Input: part model. Units: mm. Frame: model coordinates. Face numbers are marked on the shaded views. A direction names the side the tool comes from. Coordinates: 2 decimals unless noted, no trailing zeros. Write each loop counter-clockwise with the first axis right and the second up, starting at its lowest first coordinate (ties: lowest second). Pieces come first, ordered by that corner, then holes. Notation, with made-up numbers: M 61,39 L 81,39 A11 ccw 81,50 Z; hole C -1,49.5 d11. An arc over 180 degrees is marked long. Answer as a JSON object with one key per item and string values. Group by question number.
from build123d import *

# Parameters (mm, degrees)
ESBO_O1_R                     = 40
ESBO_O1_R_2                   = 30
RESSALTO_EXTRUS_O1_DEPTH      = 50
ESBO_O2_R                     = 1.5
CORTE_EXTRUS_O1_DEPTH         = 6
CORTE_EXTRUS_O2_DEPTH         = 11.84997677
RESSALTO_EXTRUS_O2_DEPTH      = 26.84997677
RESSALTO_EXTRUS_O2_DEPTH_BACK = 10
REVOLU_O1_ANGLE               = 180
RESSALTO_EXTRUS_O5_DEPTH      = 5
RESSALTO_EXTRUS_O5_DEPTH_BACK = 2
ESBO_O10_R                    = 11
ESBO_O13_R                    = 8
CORTE_EXTRUS_O4_DEPTH         = 40


# Read off the part's stored shape, not the designer's step: Limites1
with BuildPart() as part:
    # Esboço1 → Ressalto-extrusão1 (new body)
    with BuildSketch(Plane(origin=(0, 0, 0), x_dir=(1, 0, 0), z_dir=(0, 1, 0))):
        with Locations(Location((0, 0, 0), (0, 0, 270))):
            Circle(ESBO_O1_R)
        with Locations(Location((0, 0, 0), (0, 0, 270))):
            Circle(ESBO_O1_R_2, mode=Mode.SUBTRACT)
    extrude(amount=RESSALTO_EXTRUS_O1_DEPTH)

    # Esboço2 → Corte-extrusão1 (cut)
    with BuildSketch(Plane(origin=(0, 0, 0), x_dir=(-1, 0, 0), z_dir=(0, -1, 0))):
        with Locations(Location((-21.160269083, -29.124611797, 0), (0, 0, 90))):
            Circle(ESBO_O2_R)
        with Locations(Location((-34.238034587, -11.124611797, 0), (0, 0, 90))):
            Circle(ESBO_O2_R)
        with Locations(Location((-34.238034587, 11.124611797, 0), (0, 0, 90))):
            Circle(ESBO_O2_R)
        with Locations(Location((21.160269083, 29.124611797, 0), (0, 0, 90))):
            Circle(ESBO_O2_R)
        with Locations(Location((34.238034587, 11.124611797, 0), (0, 0, 90))):
            Circle(ESBO_O2_R)
        with Locations(Location((34.238034587, -11.124611797, 0), (0, 0, 90))):
            Circle(ESBO_O2_R)
    extrude(amount=-CORTE_EXTRUS_O1_DEPTH, mode=Mode.SUBTRACT)

    # Esboço3 → Corte-extrusão2 (cut)
    with BuildSketch(Plane(origin=(0, 0, 0), x_dir=(-1, 0, 0), z_dir=(0, -1, 0))):
        with BuildLine():
            ThreePointArc((30.293924668, -13.087327008), (31.253408489, 10.593604572), (16.092357529, 28.81034587))
            Line((16.092357529, 28.81034587), (19.505887914, 34.921631358))
            ThreePointArc((19.505887914, 34.921631358), (8.030354378, 39.185627576), (-4.197370073, 39.779166463))
            Line((-4.197370073, 39.779166463), (-3.148027555, 29.834374847))
            ThreePointArc((-3.148027555, 29.834374847), (29.911212101, 2.306380417), (1.462902849, -29.964310692))
            Line((1.462902849, -29.964310692), (1.950537132, -39.952414256))
            ThreePointArc((1.950537132, -39.952414256), (22.185986252, -33.283359416), (36.126859334, -17.171197823))
            Line((36.126859334, -17.171197823), (30.293924668, -13.087327008))
        make_face()
    extrude(amount=-CORTE_EXTRUS_O2_DEPTH, mode=Mode.SUBTRACT)

    # Esboço4 → Ressalto-extrusão2 (add, two sides: drawn at the far end of the back side and taken through both)
    with BuildSketch(Plane(origin=(0, 11.84997677, 0), x_dir=(-1, 0, 0), z_dir=(0, -1, 0)).offset(-RESSALTO_EXTRUS_O2_DEPTH_BACK)):
        with BuildLine():
            Line((-4.008838629, -29.730947056), (-4.700362463, -27.602655537))
            ThreePointArc((-4.700362463, -27.602655537), (-8.119302432, 26.79695744), (19.230258499, -20.351834268))
            Line((19.230258499, -20.351834268), (19.909240802, -22.441526924))
            ThreePointArc((19.909240802, -22.441526924), (-8.745833796, 28.696870757), (-4.008838629, -29.730947056))
        make_face()
    extrude(amount=RESSALTO_EXTRUS_O2_DEPTH + RESSALTO_EXTRUS_O2_DEPTH_BACK)

    # Esboço9 → Revolução1 (revolve)
    with BuildSketch(Plane(origin=(0, 50, 0), x_dir=(1, 0, 0), z_dir=(0, 1, 0))):
        with BuildLine():
            Line((-40, 0), (-30, 0))
            ThreePointArc((-30, 0), (0, 30), (30, 0))
            Line((30, 0), (40, 0))
            ThreePointArc((40, 0), (0, 40), (-40, 0))
        make_face()
    revolve(axis=Axis((-40, 50, 0), (1, 0, 0)), revolution_arc=REVOLU_O1_ANGLE)

    # Esboço10 → Ressalto-extrusão5 (add, two sides: drawn at the far end of the back side and taken through both)
    with BuildSketch(Plane(origin=(0, 90, 0), x_dir=(1, 0, 0), z_dir=(0, 1, 0)).offset(-RESSALTO_EXTRUS_O5_DEPTH_BACK)):
        with Locations(Location((0, 0, 0), (0, 0, 270))):
            Circle(ESBO_O10_R)
    extrude(amount=RESSALTO_EXTRUS_O5_DEPTH + RESSALTO_EXTRUS_O5_DEPTH_BACK)

    # Limites1 outline → Limites1 (revolve)
    with BuildSketch(Plane.XY):
        Polygon((11, 95), (10.5, 115), (0, 115), (0, 95), align=None)
    revolve(axis=Axis((0, 0, 0), (0, 1, 0)))

    # Esboço13 → Corte-extrusão4 (cut)
    with BuildSketch(Plane(origin=(0, 115, 0), x_dir=(1, 0, 0), z_dir=(0, 1, 0))):
        with Locations(Location((0, 0, 0), (0, 0, 270))):
            Circle(ESBO_O13_R)
    extrude(amount=-CORTE_EXTRUS_O4_DEPTH, mode=Mode.SUBTRACT)


solid = part.part
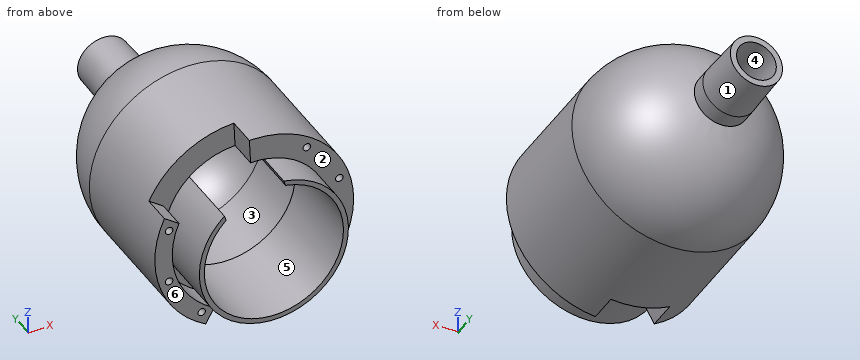
Q1. Section A-A, the plane z = 0. Return the cut outline in (x, y).
Q2. Section D-D, the plane z = -32.5. Return the cut outline in (x, y), and give its area (3 significant figures).
Q3. Section C-C, the plane y = 29. Return the cut outline in (x, z), and give its area (3 significant figures).
Q4. Pin query (flat end, axial travel): pin 1 Ø2.5 at (x, z) = (33.5, -12) entering from -Y; pin 2 Ø1.5 at (x, y) = (15.5, 63) entering from -Z; pin 3 Ø3 at (y, z) = (64.5, -12) entering from -X (3 decimals); pin 4 Ø14.5 at (x, z) = (0, 0) entering from -Y. Return the tip coordinate at first contact, or that it passes through.
Q5. Section B-B, the plane x = 0. Return the cut outline in (y, z), and give its area (3 significant figures).
Q6. Access query for the marked faces 4, 5 and 6. Directions: +Z, -Z, +X, -X, +Y, -Y. A direction counts if a zero-diameter tool reaches every point of the face in a straight line with its end or side. Return the directions, or none.
Q7. Draft query along Y for the marked faces 1, 2 and 3. Return one class per face: released by +Y, released by -Y, zero draft, split by the parting line, or undercut.
Q8. Line query: line 1 (X direction, y = 1.5, z = 0); line 2 (X direction, y = 17, z = -11); line 3 (Z direction, x = 5.5, y = 106.5). Output: solid intervals per line, ascending. Write a range as from..to.
Filled in:
{
 "1": {"outline": "M -40,0 L -33,0 L -33,11.85 L -30,11.85 L -30,-15 L -28,-15 L -28,21.85 L -30,21.85 L -30,50 A30 cw -8,78.91 L -8,115 L -10.5,115 L -11,95 L -11,88.46 A40 ccw -40,50 Z; M 8,78.91 A30 cw 30,50 L 30,21.85 L 28,21.85 L 28,-15 L 30,-15 L 30,0 L 40,0 L 40,50 A40 ccw 11,88.46 L 11,95 L 10.5,115 L 8,115 Z"},
 "2": {"outline": "M -23.32,0 L -18.15,0 L -18.15,11.85 L 3.43,11.85 L 3.43,0 L 23.32,0 L 23.32,50 A23.32 ccw -23.32,50 Z", "area": "2,930 mm^2"},
 "3": {"outline": "C 0,0 d80; hole C 0,0 d60", "area": "2,200 mm^2"},
 "4": {"pin 1": "y = 0", "pin 2": "z = -34.94", "pin 3": "x = -36.055", "pin 4": "through"},
 "5": {"outline": "M -15,-30 L 11.85,-30 L 11.85,-40 L 50,-40 A40 ccw 88.46,-11 L 95,-11 L 115,-10.5 L 115,-8 L 78.91,-8 A30 cw 50,-30 L 21.85,-30 L 21.85,-28 L -15,-28 Z; M 0,30 L 50,30 A30 cw 78.91,8 L 115,8 L 115,10.5 L 95,11 L 88.46,11 A40 ccw 50,40 L 0,40 Z", "area": "2,040 mm^2"},
 "6": {"face 4": "+Y, -Y", "face 5": "-Y", "face 6": "-Z, -X, -Y"},
 "7": {"face 1": "released by +Y", "face 2": "released by -Y", "face 3": "undercut"},
 "8": {"line 1": "-40..-33, -30..-28, 28..40", "line 2": "-38.46..-25.75, 25.75..38.46", "line 3": "-9.19..-5.81, 5.81..9.19"}
}
